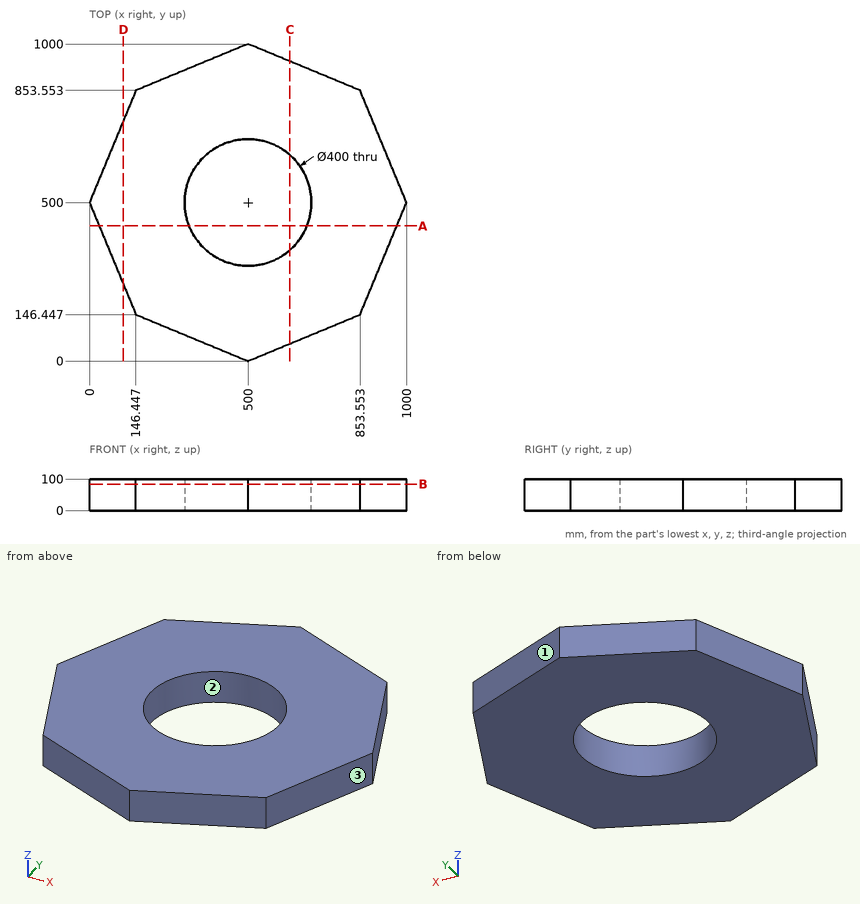
Study the drawing (mm; zero at the part's minimum x, y, z) and answer. Give positions to 0.01 mm unless a question says otherwise; leave off trailing zeros. Loops run counter-clockwise (first coordinate to the right, second up) from the corner with the lowest first, then second, coordinate; pieces in that order, holes last. Notation, with made-up numbers: (18, 50) - (65, 50) arc R24 ccw to (65, 69) - close; hole circle Ø10 at (-10, 56.25). An arc over 180 degrees is marked (long way). Answer in a Markdown table with one row per item. Add a question column.
Q1. Determine the mould class of the marked faces 1, 2 and 3 for opening direction Y: released by +Y, released by -Y, zero draft, split by the parting line, or undercut.
Q2. The part is cut by section A-A (y = 426). Determine the outline of the cut face in (x, z), and give its area (3 significant figures).
Q3. Each of these flat-tipped pins is pushed along its axis until it touches: P1, Ø12, axis at y = 420.5, z = 37.5, coming from the -X side (1 decimal); P2, Ø2, axis at y = 285.5, z = 17.5, coming from the +X side (1 decimal); P3, Ø8, axis at x = 390, z = 18.5, coming from the +Y side; P4, Ø2, axis at x = 654, y = 880.5, coming from the -Z side. Where does it stop, or does it pass through?
Q4. The part is cut by section C-C (x = 632). Determine the outline of the cut face in (y, z), and give its area (3 significant figures).
Q5. The part is cut by section B-B (z = 84). Determine the outline of the cut face in (x, y), and give its area (3 significant figures).
Q6. The part is cut by section D-D (x = 107). Determine the outline of the cut face in (y, z).
Q7. Consider line 1 along X through (y, z) = (500, 57); line 2 along X through (y, z) = (588, 42). Determine where each line is inside the solid, lowest interval first.
Solution:
| question | item | result |
|---|---|---|
| 1 | face 1 | released by +Y |
| 1 | face 2 | undercut |
| 1 | face 3 | released by -Y |
| 2 | outline | (30.65, 0) - (314.19, 0) - (314.19, 100) - (30.65, 100) - close; (685.81, 0) - (969.35, 0) - (969.35, 100) - (685.81, 100) - close |
| 2 | area | 56,700 mm² |
| 3 | P1 | stops at x = 30.4 |
| 3 | P2 | stops at x = 911.6 |
| 3 | P3 | stops at y = 956.09 |
| 3 | P4 | stops at z = 0 |
| 4 | outline | (54.68, 0) - (349.75, 0) - (349.75, 100) - (54.68, 100) - close; (650.25, 0) - (945.32, 0) - (945.32, 100) - (650.25, 100) - close |
| 4 | area | 59,000 mm² |
| 5 | outline | (0, 500) - (146.45, 146.45) - (500, 0) - (853.55, 146.45) - (1000, 500) - (853.55, 853.55) - (500, 1000) - (146.45, 853.55) - close; hole circle Ø400 at (500, 500) |
| 5 | area | 581,000 mm² |
| 6 | outline | (241.68, 0) - (758.32, 0) - (758.32, 100) - (241.68, 100) - close |
| 7 | line 1 | x = 0 to 300, 700 to 1000 |
| 7 | line 2 | x = 36.45 to 320.4, 679.6 to 963.55 |
